from build123d import *

# Parameters (mm, degrees)
CYLINDER018_R               = 2
CYLINDER018_DEPTH           = 18
CYLINDER018_PITCH_ANGLE     = 90
CYLINDER018_PLACEMENT_ANGLE = 17
BOX022_W                    = 65
BOX022_H                    = 11
BOX022_DEPTH                = 20
BOX022_PLACEMENT_ANGLE      = 15
CYLINDER017_R               = 43
CYLINDER017_DEPTH           = 19
BOX020_W                    = 10
BOX020_H                    = 21
BOX020_DEPTH                = 10


with BuildPart() as cylinder018:
    # Cylinder018 → Cylinder018 (new body)
    with BuildSketch(Plane.XY):
        Circle(CYLINDER018_R)
    extrude(amount=CYLINDER018_DEPTH)


with BuildPart() as cylinder018_1:
    # Cylinder018 pitch: moved
    add(cylinder018.part.rotate(Axis((0, 0, 0), (0, 1, 0)), CYLINDER018_PITCH_ANGLE))


with BuildPart() as cylinder018_2:
    # Cylinder018 placement: moved
    add(cylinder018_1.part.moved(Location((146.075979, 19.182766, 10))).rotate(Axis((146.075979, 19.182766, 10), (0, 0, 1)), CYLINDER018_PLACEMENT_ANGLE))


with BuildPart() as cube022:
    # Box022 → Box022 (new body)
    with BuildSketch(Plane.XY):
        with Locations((32.5, 5.5)):
            Rectangle(BOX022_W, BOX022_H)
    extrude(amount=BOX022_DEPTH)


with BuildPart() as cube022_1:
    # Box022 placement: moved
    add(cube022.part.moved(Location((115, -7, 0))).rotate(Axis((115, -7, 0), (0, 0, 1)), BOX022_PLACEMENT_ANGLE))


with BuildPart() as cylinder017:
    # Cylinder017 → Cylinder017 (new body)
    with BuildSketch(Plane(origin=(132, 63, 0), x_dir=(1, 0, 0), z_dir=(0, 0, 1))):
        Circle(CYLINDER017_R)
    extrude(amount=CYLINDER017_DEPTH)


with BuildPart() as cut028:
    # Box020 → Box020 (new body)
    with BuildSketch(Plane(origin=(151, 12, 5), x_dir=(1, 0, 0), z_dir=(0, 0, 1))):
        with Locations((5, 10.5)):
            Rectangle(BOX020_W, BOX020_H)
    extrude(amount=BOX020_DEPTH)

    # Cut026: cut Cylinder017
    add(cylinder017.part, mode=Mode.SUBTRACT)

    # Cut027: cut Cube022
    add(cube022_1.part, mode=Mode.SUBTRACT)

    # Cut028: cut Cylinder018
    add(cylinder018_2.part, mode=Mode.SUBTRACT)


solid = cut028.part
Design review of the part built by this model. Coordinates are the model's own, in mm. Round coordinates to 2 decimals unless told otherwise and drop trailing zeros. Write each loop counter-clockwise with the first axis right and the second up, starting at its lowest first coordinate (ties: lowest second). Pieces come first, ordered by that corner, then holes. Notation, with made-up numbers: (-39, 52.5) -> (4, 52.5) arc R20 cw to (4, 72.5) -> close; hole circle Ø4 at (28, 17.25). An arc over 180 degrees is marked (long way). One line per item, written item: value. Start each with the question number.
Q1. To check wall thickness, follow probe 1 along Y at (x, z) = (155, 11.25); probe 2 along Y at (x, z) = (159, 8.5); probe 3 along Z at (x, y) = (155, 21.75). State the ranges of each line that lie inside material, in increasing order.
Q2. Add section B-B (z = 7.25). Give the boundary of the cut face in (x, y).
Q3. The part is to be moulded in two halves that separate along X. For faces 1 (the face through (151, 18, 10)), 2 (the face through (155.427, 23.805, 8.925)), 3 (the face through (161, 23.9, 7.7)), say which applies: pulls with the +X half, pulls with the -X half, needs draft (parallel to the pull), parting line crosses it, or undercut.
Q4. Insertion check: P1, Ø3, axis at x = 158, z = 9, coming from the -Y side. The pin has a flat end and moves straight along its axis. Give the tip position at first contact, or say it passes through.
Q5. Add section A-A (z = 9.25). Give the boundary of the cut face in (x, y), then the cut area to 3 significant figures.
Q6. Add section C-C (y = 28.25). Give the boundary of the cut face in (x, z), then the cut area to 3 significant figures.
Response:
1. probe 1: y = 15.11 to 20.28, 23.54 to 26.67
1. probe 2: y = 16.18 to 21.75, 24.52 to 29.53
1. probe 3: z = 5 to 8.01, 11.99 to 15
2. outline: (151, 14.03) -> (161, 16.71) -> (161, 31.25) arc R43 cw to (151, 24.43) -> close
3. face 1: pulls with the -X half
3. face 2: undercut
3. face 3: pulls with the +X half
4. P1: stops at y = 15.51
5. outline: (151, 14.03) -> (161, 16.71) -> (161, 21.81) -> (151, 18.75) -> close; (151, 22.63) -> (161, 25.68) -> (161, 31.25) arc R43 cw to (151, 24.43) -> close
5. area: 82.4 mm^2
6. outline: (157.33, 5) -> (161, 5) -> (161, 15) -> (157.33, 15) -> close
6. area: 36.7 mm^2
